For this review, take the finished solid that the model builds, in its own axes (mm). Face numbers are marked on the shaded views. A direction names the side the tool comes from. Round coordinates to 2 decimals unless told otherwise and drop trailing zeros. Write each loop counter-clockwise with the first axis right and the second up, starting at its lowest first coordinate (ties: lowest second). Pieces come first, ordered by that corner, then holes. Notation, with made-up numbers: (51.5, 47.25) - (74.5, 47.25) arc R22 cw to (74.5, 63.25) - close; hole circle Ø5 at (-30, -35). An arc over 180 degrees is marked (long way). One line per item, written item: value. Start each with the question number.
Q1. Mouldability with a two-part tool opening along X and no side actions: class the marked faces 1, 2, 3 and 4 as +X half, -X half, draft (parallel to the pull), parting line (faces both ways), or undercut.
Q2. Add section C-C on y = -3.5. Write out the cut boundary in (x, z), and give its area (3 significant figures).
Q3. Add section D-D on x = -20.5. Write out the cut boundary in (y, z).
Q4. Add section B-B on x = 10.5. Write out the cut boundary in (y, z), and give its area (3 significant figures).
Q5. For probe 1 along Y at (x, z) = (20.5, 1.8); probe 2 along X at (y, z) = (14, -11.75); probe 3 along Y at (x, z) = (-10.5, 2.5), list the stretches that pass through material, from the lowest coordinate up.
Q6. Tool access review of the marked faces 5, 6, 7 and 8: name each direction out of +Z, -Z, +X, -X, +Y, -Y from which nothing blocks a thin tool from reaching the whole face with its end or side.
Q7. Add section A-A on z = -7.25. Write out the cut boundary in (x, y) (3 decimals).
Q8. Clearance check with flat-ended pins moving along their axes: pin 1 Ø3 at (y, z) = (3, -3.5) entering from -X; pin 2 Ø4 at (x, y) = (20.5, 28) entering from +Z; pin 3 Ø1.5 at (x, y) = (5.5, -9.5) entering from -Z. State where each tip first meets the part, or that it passes through.
```python
from build123d import *

# Parameters (mm, degrees)
SKIZZE1_R                        = 3
AUFSATZ_KAMERA_HALTERUNG_DEPTH   = 3
AUFSATZ_KAMERA_HALTERUNG_2_DEPTH = 3
AUFSATZ_KAMERA_HALTERUNG_3_DEPTH = 3
AUFSATZ_KAMERA_HALTERUNG_4_DEPTH = 3
SKIZZE2_W                        = 43
SKIZZE2_H                        = 40
DECKEL_DEPTH                     = 3
SKIZZE3_R                        = 1.7
L_CHER_KAMERA_HALTERUNG_DEPTH    = 4
SKIZZE4_W                        = 49
SKIZZE4_H                        = 45.581395348
SKIZZE4_W_2                      = 43
SKIZZE4_H_2                      = 40
AUFSATZ_LINEAR_AUSTRAGEN1_DEPTH  = 27
SKIZZE6_W                        = 25
SKIZZE6_H                        = 3
SCHNITT_LINEAR_AUSTRAGEN1_DEPTH  = 2.790698
SKIZZE7_R                        = 4
AUFSATZ_LINEAR_AUSTRAGEN2_DEPTH  = 27
SKIZZE8_R                        = 2.1
SCHNITT_LINEAR_AUSTRAGEN2_DEPTH  = 5.7
SKIZZE9_W                        = 0.18718111
SKIZZE9_H                        = 1.209302326
AUFSATZ_LINEAR_AUSTRAGEN3_DEPTH  = 27
SKIZZE10_R                       = 2.1
SCHNITT_LINEAR_AUSTRAGEN3_DEPTH  = 5.7
SKIZZE11_R                       = 3
AUFSATZ_LINEAR_AUSTRAGEN4_DEPTH  = 6
SKIZZE12_R                       = 1.7
SCHNITT_LINEAR_AUSTRAGEN4_DEPTH  = 4
FASE1_SIZE                       = 2
FASE1_SIZE2                      = 5.494954839


with BuildPart() as part:
    # Skizze1 → Aufsatz Kamera Halterung (new body)
    with BuildSketch(Plane.XY):
        with Locations((10.5, -3.5)):
            Circle(SKIZZE1_R)
    extrude(amount=AUFSATZ_KAMERA_HALTERUNG_DEPTH)



with BuildPart() as body_2:
    # Skizze1 → Aufsatz Kamera Halterung 2 (new body)
    with BuildSketch(Plane.XY):
        with Locations((10.5, 10)):
            Circle(SKIZZE1_R)
    extrude(amount=AUFSATZ_KAMERA_HALTERUNG_2_DEPTH)


with BuildPart() as body_3:
    # Skizze1 → Aufsatz Kamera Halterung 3 (new body)
    with BuildSketch(Plane.XY):
        with Locations((-10.5, 10)):
            Circle(SKIZZE1_R)
    extrude(amount=AUFSATZ_KAMERA_HALTERUNG_3_DEPTH)


with BuildPart() as body_4:
    # Skizze1 → Aufsatz Kamera Halterung 4 (new body)
    with BuildSketch(Plane.XY):
        with Locations((-10.5, -3.5)):
            Circle(SKIZZE1_R)
    extrude(amount=AUFSATZ_KAMERA_HALTERUNG_4_DEPTH)


with BuildPart() as part_1:
    add(part.part)

    add(body_2.part)  # Deckel merges body 2

    add(body_3.part)  # Deckel merges body 3

    add(body_4.part)  # Deckel merges body 4
    # Skizze2 → Deckel (add)
    with BuildSketch(Plane.XY.offset(3)):
        with Locations((0, 4)):
            Rectangle(SKIZZE2_W, SKIZZE2_H)
    extrude(amount=DECKEL_DEPTH)

    # Skizze3 → Löcher Kamera Halterung (cut)
    with BuildSketch(Plane(origin=(0, 0, 0), x_dir=(-1, 0, 0), z_dir=(0, 0, -1))):
        with Locations((10.5, 10)):
            Circle(SKIZZE3_R)
        with Locations((10.5, -3.5)):
            Circle(SKIZZE3_R)
        with Locations((-10.5, -3.5)):
            Circle(SKIZZE3_R)
        with Locations((-10.5, 10)):
            Circle(SKIZZE3_R)
    extrude(amount=-L_CHER_KAMERA_HALTERUNG_DEPTH, mode=Mode.SUBTRACT)

    # Skizze4 → Aufsatz-Linear austragen1 (add)
    with BuildSketch(Plane.XY.offset(6)):
        with Locations((0, 4)):
            Rectangle(SKIZZE4_W, SKIZZE4_H)
        with Locations((0, 4)):
            Rectangle(SKIZZE4_W_2, SKIZZE4_H_2, mode=Mode.SUBTRACT)
    extrude(amount=-AUFSATZ_LINEAR_AUSTRAGEN1_DEPTH)

    # Skizze6 → Schnitt-Linear austragen1 (cut)
    with BuildSketch(Plane(origin=(0, -18.790697674, 0), x_dir=(-1, 0, 0), z_dir=(0, -1, 0))):
        with Locations((0, 2)):
            Rectangle(SKIZZE6_W, SKIZZE6_H)
    extrude(amount=-SCHNITT_LINEAR_AUSTRAGEN1_DEPTH, mode=Mode.SUBTRACT)

    # Skizze7 → Aufsatz-Linear austragen2 (add, through all)
    with BuildSketch(Plane(origin=(0, 0, -21), x_dir=(-1, 0, 0), z_dir=(0, 0, -1))):
        with Locations((-20.5, 28)):
            Circle(SKIZZE7_R)
        with Locations((20.5, 28)):
            Circle(SKIZZE7_R)
        with Locations((20.5, -20)):
            Circle(SKIZZE7_R)
        with Locations((-20.5, -20)):
            Circle(SKIZZE7_R)
    extrude(amount=-AUFSATZ_LINEAR_AUSTRAGEN2_DEPTH)

    # Skizze8 → Schnitt-Linear austragen2 (cut)
    with BuildSketch(Plane(origin=(0, 0, -21), x_dir=(-1, 0, 0), z_dir=(0, 0, -1))):
        with Locations((-20.5, 28)):
            Circle(SKIZZE8_R)
        with Locations((20.5, 28)):
            Circle(SKIZZE8_R)
        with Locations((20.5, -20)):
            Circle(SKIZZE8_R)
        with Locations((-20.5, -20)):
            Circle(SKIZZE8_R)
    extrude(amount=-SCHNITT_LINEAR_AUSTRAGEN2_DEPTH, mode=Mode.SUBTRACT)

    # Skizze9 → Aufsatz-Linear austragen3 (add, through all)
    with BuildSketch(Plane(origin=(0, 0, -21), x_dir=(-1, 0, 0), z_dir=(0, 0, -1))):
        with Locations((-24.406409445, 27.395348837)):
            Rectangle(SKIZZE9_W, SKIZZE9_H)
        with Locations((24.406409445, 27.395348837)):
            Rectangle(SKIZZE9_W, SKIZZE9_H)
        with Locations((24.406409445, -19.395348837)):
            Rectangle(SKIZZE9_W, SKIZZE9_H)
        with Locations((-24.406409445, -19.395348837)):
            Rectangle(SKIZZE9_W, SKIZZE9_H)
        with BuildLine():
            Line((-18.024994038, 31.142347131), (-12.5, 26.790697674))
            Line((-12.5, 26.790697674), (-16.68718111, 26.790697674))
            ThreePointArc((-16.68718111, 26.790697674), (-16.676598558, 29.175415421), (-18.024994038, 31.142347131))
        make_face()
        with BuildLine():
            Line((12.5, 26.790697674), (16.68718111, 26.790697674))
            ThreePointArc((16.68718111, 26.790697674), (16.676598558, 29.175415421), (18.024994038, 31.142347131))
            Line((18.024994038, 31.142347131), (12.5, 26.790697674))
        make_face()
        with BuildLine():
            Line((18.024994038, -23.142347131), (12.5, -18.790697674))
            Line((12.5, -18.790697674), (16.68718111, -18.790697674))
            ThreePointArc((16.68718111, -18.790697674), (16.676598558, -21.175415421), (18.024994038, -23.142347131))
        make_face()
        with BuildLine():
            Line((-12.5, -18.790697674), (-16.68718111, -18.790697674))
            ThreePointArc((-16.68718111, -18.790697674), (-16.676598558, -21.175415421), (-18.024994038, -23.142347131))
            Line((-18.024994038, -23.142347131), (-12.5, -18.790697674))
        make_face()
    extrude(amount=-AUFSATZ_LINEAR_AUSTRAGEN3_DEPTH)

    # Skizze10 → Schnitt-Linear austragen3 (cut)
    with BuildSketch(Plane.XY.offset(6)):
        with Locations((-20.5, 28)):
            Circle(SKIZZE10_R)
        with Locations((20.5, 28)):
            Circle(SKIZZE10_R)
        with Locations((20.5, -20)):
            Circle(SKIZZE10_R)
        with Locations((-20.5, -20)):
            Circle(SKIZZE10_R)
    extrude(amount=-SCHNITT_LINEAR_AUSTRAGEN3_DEPTH, mode=Mode.SUBTRACT)

    # Skizze11 → Aufsatz-Linear austragen4 (add)
    with BuildSketch(Plane.ZY.offset(24.5)):
        with Locations((-15.2, -14.85)):
            Circle(SKIZZE11_R)
    extrude(amount=AUFSATZ_LINEAR_AUSTRAGEN4_DEPTH)

    # Skizze12 → Schnitt-Linear austragen4 (cut)
    with BuildSketch(Plane.ZY.offset(30.5)):
        with Locations((-15.2, -14.85)):
            Circle(SKIZZE12_R)
    extrude(amount=-SCHNITT_LINEAR_AUSTRAGEN4_DEPTH, mode=Mode.SUBTRACT)

    # Fase1
    fase1_edges = [part_1.edges().sort_by_distance(p)[0] for p in [
        (-24.5, -14.85, -18.2),
    ]]
    fase1_side = [part_1.faces().sort_by_distance(p)[0] for p in [
        (-24.5, 4.443247545, -7.318938669),
    ]]
    chamfer(fase1_edges, length=FASE1_SIZE, length2=FASE1_SIZE2, reference=fase1_side[0])


solid = part_1.part
```
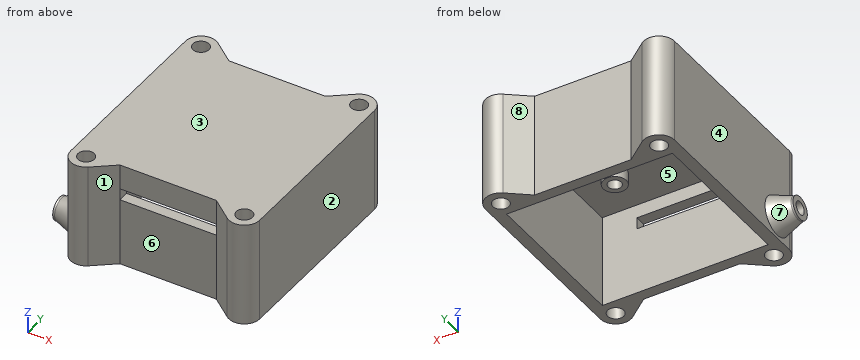
Result set:
1. face 1: undercut
1. face 2: +X half
1. face 3: draft
1. face 4: -X half
2. outline: (-24.5, -21) - (-21.5, -21) - (-21.5, 3) - (-13.5, 3) - (-13.5, 0) - (-12.2, 0) - (-12.2, 4) - (-8.8, 4) - (-8.8, 0) - (-7.5, 0) - (-7.5, 3) - (7.5, 3) - (7.5, 0) - (8.8, 0) - (8.8, 4) - (12.2, 4) - (12.2, 0) - (13.5, 0) - (13.5, 3) - (21.5, 3) - (21.5, -21) - (24.5, -21) - (24.5, 6) - (-24.5, 6) - close
2. area: 300 mm^2
3. outline: (-24, -21) - (-22.1, -21) - (-22.1, -15.3) - (-17.9, -15.3) - (-17.9, -21) - (-16, -21) - (-16, 3) - (24, 3) - (24, -21) - (25.9, -21) - (25.9, -15.3) - (30.1, -15.3) - (30.1, -21) - (32, -21) - (32, 6) - (30.1, 6) - (30.1, 0.3) - (25.9, 0.3) - (25.9, 6) - (-17.9, 6) - (-17.9, 0.3) - (-22.1, 0.3) - (-22.1, 6) - (-24, 6) - close
4. outline: (-18.79, -21) - (-16, -21) - (-16, -3.5) - (-18.79, -3.5) - close; (-18.79, -0.5) - (-16, -0.5) - (-16, 3) - (-6.5, 3) - (-6.5, 0) - (-5.2, 0) - (-5.2, 4) - (-1.8, 4) - (-1.8, 0) - (-0.5, 0) - (-0.5, 3) - (7, 3) - (7, 0) - (8.3, 0) - (8.3, 4) - (11.7, 4) - (11.7, 0) - (13, 0) - (13, 3) - (24, 3) - (24, -21) - (26.79, -21) - (26.79, 6) - (-18.79, 6) - close
4. area: 271 mm^2
5. probe 1: y = -24 to -22.1, -17.9 to -16, 24 to 25.9, 30.1 to 32
5. probe 2: x = -24.5 to -21.5, 21.5 to 24.5
5. probe 3: y = -18.79 to -16, -6.5 to -5.2, -1.8 to -0.5, 7 to 8.3, 11.7 to 13, 24 to 26.79
6. face 5: -Z
6. face 6: +Z, -Z, -Y
6. face 7: -X
6. face 8: +Z, -Z, +Y
7. outline: (-24.5, -20) arc R4 ccw to (-18.025, -23.142) - (-12.5, -18.791) - (12.5, -18.791) - (18.025, -23.142) arc R4 ccw to (24.5, -20) - (24.5, 28) arc R4 ccw to (18.025, 31.142) - (12.5, 26.791) - (-12.5, 26.791) - (-18.025, 31.142) arc R4 ccw to (-24.5, 28) - close; hole (-21.5, -16) - (21.5, -16) - (21.5, 24) - (-21.5, 24) - close
8. pin 1: stops at x = -24.5
8. pin 2: stops at z = 0.3
8. pin 3: stops at z = 3
